from build123d import *

# Parameters (mm, degrees)
EXTRUDE_1_DEPTH     = 4
SKETCH_4_R          = 1.5
CUT_EXTRUDE_1_DEPTH = 15
SKETCH_3_R          = 7
EXTRUDE_4_DEPTH     = 2
SKETCH_10_R         = 5
EXTRUDE_7_DEPTH     = 4
SKETCH_11_R         = 7
EXTRUDE_8_DEPTH     = 2
SKETCH_12_R         = 4
CUT_EXTRUDE_5_DEPTH = 4


with BuildPart() as part:
    # 草图2 → 凸台-拉伸1 (new body)
    with BuildSketch(Plane(origin=(0, 0, 0), x_dir=(1, 0, 0), z_dir=(0, 1, 0))):
        Polygon((0, 0), (-2.5, 4.330127019), (-5, 0), align=None)
        Polygon((-2.5, -4.330127019), (-5, 0), (0, 0), align=None)
        Polygon((0, 0), (-2.5, -4.330127019), (2.5, -4.330127019), align=None)
        Polygon((0, 0), (2.5, -4.330127019), (5, 0), align=None)
        Polygon((0, 0), (5, 0), (2.5, 4.330127019), align=None)
        Polygon((0, 0), (2.5, 4.330127019), (-2.5, 4.330127019), align=None)
    extrude(amount=EXTRUDE_1_DEPTH)

    # 草图4 → 切除-拉伸1 (cut)
    with BuildSketch(Plane.XZ):
        with Locations(Location((0, 0, 0), (0, 0, 270))):
            Circle(SKETCH_4_R)
    extrude(amount=-CUT_EXTRUDE_1_DEPTH, mode=Mode.SUBTRACT)

    # 草图3 → 凸台-拉伸4 (add)
    with BuildSketch(Plane(origin=(0, 4, 0), x_dir=(1, 0, 0), z_dir=(0, 1, 0))):
        with Locations(Location((0, 0, 0), (0, 0, 270))):
            Circle(SKETCH_3_R)
    extrude(amount=EXTRUDE_4_DEPTH)

    # 草图10 → 凸台-拉伸7 (add)
    with BuildSketch(Plane(origin=(0, 6, 0), x_dir=(1, 0, 0), z_dir=(0, 1, 0))):
        with Locations(Location((0, 0, 0), (0, 0, 270))):
            Circle(SKETCH_10_R)
    extrude(amount=EXTRUDE_7_DEPTH)

    # 草图11 → 凸台-拉伸8 (add)
    with BuildSketch(Plane(origin=(0, 10, 0), x_dir=(1, 0, 0), z_dir=(0, 1, 0))):
        with Locations(Location((0, 0, 0), (0, 0, 270))):
            Circle(SKETCH_11_R)
    extrude(amount=EXTRUDE_8_DEPTH)

    # 草图12 → 切除-拉伸5 (cut)
    with BuildSketch(Plane(origin=(0, 12, 0), x_dir=(1, 0, 0), z_dir=(0, 1, 0))):
        with Locations(Location((0, 0, 0), (0, 0, 270))):
            Circle(SKETCH_12_R)
    extrude(amount=-CUT_EXTRUDE_5_DEPTH, mode=Mode.SUBTRACT)


solid = part.part
Input: part model. Units: mm. Frame: model coordinates. A direction names the side the tool comes from. Coordinates: 2 decimals unless noted, no trailing zeros. Loops run counter-clockwise (first coordinate to the right, second up) from the corner with the lowest first, then second, coordinate; pieces in that order, holes last.
Q1. Contact query for flat-ended pins moving along their axis: pin 1 (2.5 mm diameter, centred on x = 0, z = 0, fed in from -Y); pin 2 (1.2 mm diameter, centred on x = -1, y = 2, fed in from -Z); pin 3 (5 mm diameter, centred on x = 0, z = 0, fed in from +Y). Output: stop coordinate, or through.
Q2. Cut plane C-C (z = 6). Output: boundary loops of the cut face in (x, y), then the cut area to 3 significant figures.
Q3. Draft query along X for faces 1 (the face through (0, 4, 0)), 2 (the face through (3.73, 1.97, 2.2)), 3 (the face through (-6.834, 10.986, -1.517)). Return one class per face: +X half, -X half, draft (parallel to the pull), parting line (faces both ways), or undercut.
Q4. Cut plane B-B (y = 3.75). Output: boundary loops of the cut face in (x, z).
Q5. Set-up query: faces 4 (the face through (-3.905, 10.028, -0.867)), 5 (the face through (0, 2, -4.33)), 6 (the face through (3.77, 1.97, -2.13)), 7 (the face through (0, 2, 4.33)), 8 (the face through (-4.88, 7.97, -1.08)). Return all of +Z, -Z, +X, -X, +Y, -Y with unobstructed straight access to the full face (end or side cutting, diameter ignored); none if empty.
Q6. Material intervals for line 1 (X direction, y = 9.5, z = 0); line 2 (Y direction, x = -4.5, z = -3); line 3 (Z direction, x = 3, y = 6.5), sorted ascending.
Q7. Cut plane D-D (x = 0). Output: boundary loops of the cut face in (y, z), then the cut area to 3 significant figures.
Q8. Cut plane A-A (x = 5.5). Output: boundary loops of the cut face in (y, z).
Working result:
1. pin 1: stops at y = 4
1. pin 2: stops at z = -4.33
1. pin 3: stops at y = 8
2. outline: (-3.61, 4) - (3.61, 4) - (3.61, 6) - (-3.61, 6) - close; (-3.61, 10) - (3.61, 10) - (3.61, 12) - (-3.61, 12) - close
2. area: 28.8 mm2
3. face 1: undercut
3. face 2: +X half
3. face 3: parting line
4. outline: (-5, 0) - (-2.5, -4.33) - (2.5, -4.33) - (5, 0) - (2.5, 4.33) - (-2.5, 4.33) - close; hole circle Ø3 at (0, 0)
5. face 4: +Y
5. face 5: -Z, +X, -X, -Y
5. face 6: -Z, +X, -Y
5. face 7: +Z, +X, -X, -Y
5. face 8: none
6. line 1: x = -5 to -4, 4 to 5
6. line 2: y = 4 to 6, 10 to 12
6. line 3: z = -4 to 4
7. outline: (0, -4.33) - (4, -4.33) - (4, -7) - (6, -7) - (6, -5) - (10, -5) - (10, -7) - (12, -7) - (12, -4) - (8, -4) - (8, 4) - (12, 4) - (12, 7) - (10, 7) - (10, 5) - (6, 5) - (6, 7) - (4, 7) - (4, 4.33) - (0, 4.33) - (0, 1.5) - (4, 1.5) - (4, -1.5) - (0, -1.5) - close
7. area: 86.6 mm2
8. outline: (4, -4.33) - (6, -4.33) - (6, 4.33) - (4, 4.33) - close; (10, -4.33) - (12, -4.33) - (12, 4.33) - (10, 4.33) - close
